Autodesk Fusion 360 part; units mm, degrees
sketch "Skizze1" plane through (0, 0, 0) normal (0, 1, 0) x (1, 0, 0)
  line L0 (-26.8409, 12.6917) -> (1.6591, 12.6917)
  line L1 (1.6591, 12.6917) -> (1.6591, -0.8083)
  line L2 (1.6591, -0.8083) -> (-26.8409, -0.8083)
  line L3 (-26.8409, -0.8083) -> (-26.8409, 12.6917)
  line L4 (-28.8409, 14.6917) -> (3.6591, 14.6917)
  line L5 (3.6591, 14.6917) -> (3.6591, -3.8083)
  line L6 (3.6591, -3.8083) -> (-28.8409, -3.8083)
  line L7 (-28.8409, -3.8083) -> (-28.8409, 14.6917)
  line L8 (-21.3409, 10.6917) -> (-3.8409, 10.6917)
  line L9 (-3.8409, 10.6917) -> (-3.8409, 1.6917)
  line L10 (-3.8409, 1.6917) -> (-21.3409, 1.6917)
  line L11 (-21.3409, 1.6917) -> (-21.3409, 10.6917)
  dimension "d1" = 28.5
  dimension "d2" = 13.5
  dimension "d3" = 2
  dimension "d4" = 3
  dimension "d5" = 2
  dimension "d6" = 2
  dimension "d8" = 5.5
  dimension "d9" = 5.5
  dimension "d10" = 2
  dimension "d11" = 2.5
extrude "Extrusion1" add sketch "Skizze1" along normal blind 35 contours L4 L5 L6 L7
extrude "Extrusion2" add sketch "Skizze1" against normal blind 1 contours L0 L1 L2 L3 | L4 L5 L6 L7
sketch "Skizze2" plane through (0, 0, -14.6917) normal (0, 0, -1) x (-1, 0, 0)
  line L0 (28.8409, -1) -> (28.8409, 35)
  line L1 (28.8409, 35) -> (-3.6591, 35)
  line L2 (-3.6591, 35) -> (-3.6591, -1)
  line L3 (-3.6591, -1) -> (28.8409, -1)
  line L4 (6.3409, 35) -> (18.8409, 35)
  line L5 (18.8409, 35) -> (18.8409, 5)
  line L6 (18.8409, 5) -> (6.3409, 5)
  line L7 (6.3409, 5) -> (6.3409, 35)
  line L8 (28.8409, 0) -> (-3.6591, 0)
  dimension "d16" = 10
  dimension "d17" = 10
  dimension "d18" = 5
extrude "Extrusion3" cut sketch "Skizze2" against normal blind 2 contours L1 L4 L5 L6 L7
fillet "Abrundung1" radius 6 4 edges at (-6.3409, 35, -13.6917) (-18.8409, 35, -13.6917) (-18.8409, 5, -13.6917) (-6.3409, 5, -13.6917)
fillet "Abrundung2" radius 1 43 edges at (-28.8409, 17, -14.6917) (-12.5909, -1, -14.6917) (-28.8409, -1, -5.4417) (3.6591, 17, -14.6917) (3.6591, -1, -5.4417) (-12.5909, -1, -1.6917) (-3.8409, -1, -6.1917) (-12.5909, -1, -10.6917) (-21.3409, -1, -6.1917) (1.6591, 35, -14.6917) (-4.5835, 33.2426, -14.6917) (-6.3409, 20, -14.6917) (-8.0983, 6.7574, -14.6917) (-12.5909, 5, -14.6917) (-17.0835, 6.7574, -14.6917) (-18.8409, 20, -14.6917) (-20.5983, 33.2426, -14.6917) (-26.8409, 35, -14.6917) (-28.8409, 35, -5.4417) (-26.8409, 35, -5.9417) (1.6591, 35, -5.9417) (-12.5909, 35, 0.8083) (3.6591, 35, -5.4417) (1.6591, 17.5, 0.8083) (-26.8409, 17.5, 0.8083) (-12.5909, 0, 0.8083) (1.6591, 17.5, -12.6917) (1.6591, 0, -5.9417) (-12.5909, 0, -12.6917) (-26.8409, 0, -5.9417) (-25.8409, 35, -12.6917) (-20.5983, 33.2426, -12.6917) (-18.8409, 20, -12.6917) (-17.0835, 6.7574, -12.6917) (-12.5909, 5, -12.6917) (-8.0983, 6.7574, -12.6917) (-6.3409, 20, -12.6917) (-4.5835, 33.2426, -12.6917) (0.6591, 35, -12.6917) (-3.8409, -0.5, -10.6917) (-21.3409, -0.5, -10.6917) (-21.3409, -0.5, -1.6917) (-3.8409, -0.5, -1.6917)
sketch "Skizze3" plane through (0, 0, 0.8083) normal (0, 0, -1) x (-1, 0, 0)
  line L0 (-0.6591, 1) -> (25.8409, 1)
  line L1 (25.8409, 1) -> (25.8409, 34)
  line L2 (25.8409, 34) -> (-0.6591, 34)
  line L3 (-0.6591, 34) -> (-0.6591, 1)
  line L4 (25.8409, 35) -> (-0.6591, 35)
  line L5 (-2.6591, 0) -> (-2.6591, 34)
  line L6 (27.8409, 34) -> (27.8409, 0)
  point P0 (12.5909, 27)
  dimension "d25" = 8
  dimension "d26" = 15.25
  dimension "d27" = 15.25
hole "Bohrung1" at (-12.5909, 27, 0.8083) direction (0, 0, 1) diameter 4.5 depth 25 tip angle 118 countersink diameter 9 countersink angle 90
equation "d5 = d3"
equation "d6 = d3"
equation "d17 = d16"
Build history of the part. All positions in model axes, mm. A direction names the side the tool comes from. Round coordinates to 2 decimals unless told otherwise and drop trailing zeros. Answer in a Markdown table with one row per item.
1. Saw through at D-D (x = -14). State how many separate pieces and enclosed holes the cut face has, and give its area (3 significant figures).
Geometry check:
| item | result |
|---|---|
| separate pieces | 3 |
| enclosed holes | 0 |
| area | 108 mm2 |
2. Mould opens along Z. For faces 5 (the face through (-12.59, 4.71, -12.99)), 6 (the face through (-28.556, 34.699, -5.064)), 7 (the face through (1.18, 34.699, -14.407)) say: +Z half, -Z half, draft (parallel to the pull), parting line (faces both ways), or undercut.
Geometry check:
| item | result |
|---|---|
| face 5 | undercut |
| face 6 | draft |
| face 7 | -Z half |
3. Flat gauge pins, fed straight in: P1, Ø1.5, axis at x = -22, z = -10, coming from the +Y side; P2, Ø10, axis at x = -3.5, z = -6.5, coming from the +Y side. Where does each tip first touch, or does it go through?
Geometry check:
| item | result |
|---|---|
| P1 | y = 0 |
| P2 | y = 0.46 |
4. Which spindle directions (+Z, -Z, +X, -X, +Y, -Y) get a long thin tool onto all of the face, cutting with end or side? Do faces 1 (the face through (-12.48, -0.7, -10.98)), 2 (the face through (-12.587, 4.699, -14.407)), 3 (the face through (-12.776, 34.715, 1.109)), 4 (the face through (-13, -1, 1)). Say none if no direction does.
Geometry check:
| item | result |
|---|---|
| face 1 | -Y |
| face 2 | -Z, +Y |
| face 3 | +Y |
| face 4 | +Z, -Z, +X, -X, -Y |
5. Probe L1, parallel to Z at x = -4, y = 25; L2, parallel to X at y = 27, z = 3.5; L3, parallel to X at y = 18.5, z = -5.25. List the from-to ranges inside material, lowest first. Write a range as [from, to].
Geometry check:
| item | result |
|---|---|
| L1 | [-14.69, -12.69], [0.81, 3.81] |
| L2 | [-28.84, -14.84], [-10.34, 3.66] |
| L3 | [-28.84, -26.84], [1.66, 3.66] |
